Here's the drawing with two shaded views (mm, measured from the low corner). I have some questions. Give positions to 0.01 mm unless a question says otherwise; leave off trailing zeros. Loops run counter-clockwise (first coordinate to the right, second up) from the corner with the lowest first, then second, coordinate; pieces in that order, holes last. Notation, with made-up numbers: (72, 15.5) - (84, 15.5) arc R16 ccw to (84, 22.5) - close; hole circle Ø7 at (35.5, 43.25). An arc over 180 degrees is marked (long way). Use one line per item in the form item = value.
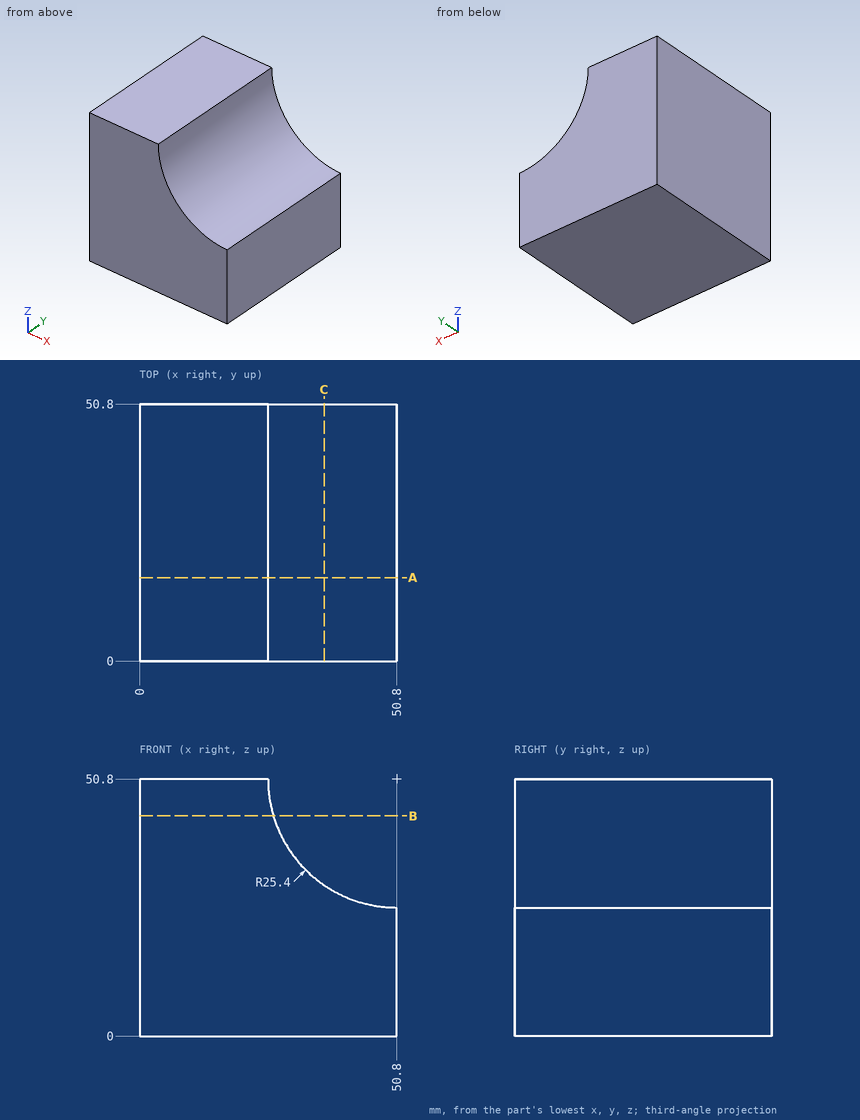
(1) For P1, Ø5, axis at x = 22, z = 44, coming from the -Y side; P2, Ø5, axis at x = 35, y = 37.5, coming from the +Z side, each with a flat end and sliding along its axis, tell me the tip position at first contact or that it passes through.
Geometry says:
P1 = 0
P2 = 33.19
(2) If we section it at C-C (x = 36.5): List the corners of the cut face in (y, z) for me, plus the area to 3 significant figures.
Geometry says:
outline = (0, 0) - (50.8, 0) - (50.8, 29.81) - (0, 29.81) - close
area = 1,510 mm²
(3) If we section it at B-B (z = 43.5): List the corners of the cut face in (x, y) for me, plus the area to 3 significant figures.
Geometry says:
outline = (0, 0) - (26.47, 0) - (26.47, 50.8) - (0, 50.8) - close
area = 1,340 mm²
(4) If we section it at A-A (y = 16.5): List the corners of the cut face in (x, z) for me.
Geometry says:
outline = (0, 0) - (50.8, 0) - (50.8, 25.4) arc R25.4 cw to (25.4, 50.8) - (0, 50.8) - close
(5) If I drill on probe 1 along X at (y, z) = (15, 35); probe 2 along X at (y, z) = (4.5, 45.5); probe 3 along Z at (x, y) = (37, 17), over which ranges is the centre line in solid material (lowest first)?
Geometry says:
probe_1 = 0 to 30.91
probe_2 = 0 to 25.96
probe_3 = 0 to 29.48
